Source: CAD feature listing. Evaluate the final solid. Frame: model axes, mm. A direction names the side the tool comes from. Coordinates: 2 decimals unless noted, no trailing zeros. Order: outer loops, then holes, each group sorted by start corner. A loop starts at its lowest first (then second) coordinate and runs counter-clockwise, first axis right, second up. Notation, with made-up numbers: (50.25, 20) -> (80.25, 20) arc R36 ccw to (80.25, 58) -> close; hole circle Ø8 at (-29, 36.25). An arc over 180 degrees is marked (long way). Write item = value, one per line. Start each with the question number.
Item 1: Section query D-D (y = -20). Output: boundary loops of the cut face in (x, z).
Item 2: Set-up query: faces 4 (the cylindrical face through (-0.521, -16.034, 2.535)), 5 (the flat face through (0, 1, 5)). Return all of +Z, -Z, +X, -X, +Y, -Y with unobstructed straight access to the full face (end or side cutting, diameter ignored); none if empty.
Item 3: Section query C-C (x = 9). Output: boundary loops of the cut face in (y, z), then the cut area to 3 significant figures.
Item 4: Contact query for flat-ended pins moving along their axis: pin 1 (1 mm diameter, centred on x = -17, y = 9.5, fed in from -Z); pin 2 (3 mm diameter, centred on x = -5, z = 42, fed in from -Y). Output: stop coordinate, or through.
Item 5: Mould query, pull axis X, two halves, no side actions, for faces 1 (the cylindrical face through (17.482, -32.871, 67.535)), 2 (the cylindrical face through (-0.521, -16.034, 67.535)), 3 (the flat face through (-6, 40, 35)). Classes: released by +X, released by -X, zero draft, split by the parting line, or undercut.
Item 6: Section query A-A (y = -5). Output: boundary loops of the cut face in (x, z), then the cut area to 3 significant figures.
Item 7: Ray query, line 1 along Z through (x, y) = (15, -21); line 2 along Y through (x, z) = (0, 1.65); line 3 along Z through (x, y) = (0, 43). Return the intervals inside material, ascending. Write a range as [from, to].
Item 8: Section query B-B (z = 35). Output: boundary loops of the cut face in (x, y).
```python
from build123d import *

# Parameters (mm, degrees)
SKETCH_1_W          = 50
SKETCH_1_H          = 80
EXTRUDE_1_DEPTH     = 5
SKETCH_2_W          = 50
SKETCH_2_H          = 80
EXTRUDE_2_DEPTH     = 5
SKETCH_3_W          = 50
SKETCH_3_H          = 70
EXTRUDE_3_DEPTH     = 5
SKETCH_4_R          = 4
CUT_EXTRUDE_1_DEPTH = 87.890735985
SKETCH_5_R          = 4
CUT_EXTRUDE_2_DEPTH = 113.915897906
FILLET_1_R          = 25


with BuildPart() as part:
    # Sketch 1 → Extrude 1 (new body)
    with BuildSketch(Plane.XY):
        Rectangle(SKETCH_1_W, SKETCH_1_H)
    extrude(amount=EXTRUDE_1_DEPTH)



with BuildPart() as body_2:
    # Sketch 2 → Extrude 2 (new body)
    with BuildSketch(Plane.XY.offset(65)):
        Rectangle(SKETCH_2_W, SKETCH_2_H)
    extrude(amount=EXTRUDE_2_DEPTH)


with BuildPart() as part_1:
    add(part.part)

    add(body_2.part)  # Extrude 3 merges body 2
    # Sketch 3 → Extrude 3 (add)
    with BuildSketch(Plane(origin=(0, 40, 0), x_dir=(1, 0, 0), z_dir=(0, 1, 0))):
        with Locations((0, -35)):
            Rectangle(SKETCH_3_W, SKETCH_3_H)
    extrude(amount=EXTRUDE_3_DEPTH)

    # Sketch 4 → Cut-Extrude 1 (cut, through all)
    with BuildSketch(Plane.XY.offset(70)):
        with Locations((0, -20)):
            Circle(SKETCH_4_R)
    extrude(amount=-CUT_EXTRUDE_1_DEPTH, mode=Mode.SUBTRACT)

    # Sketch 5 → Cut-Extrude 2 (cut, through all)
    with BuildSketch(Plane(origin=(0, 45, 0), x_dir=(1, 0, 0), z_dir=(0, 1, 0))):
        with Locations(Location((0, -35, 0), (0, 0, 180))):
            Circle(SKETCH_5_R)
    extrude(amount=-CUT_EXTRUDE_2_DEPTH, mode=Mode.SUBTRACT)

    # Fillet 1
    fillet_1_edges = [part_1.edges().sort_by_distance(p)[0] for p in [
        (-25, -40, 2.5),
        (25, -40, 2.5),
        (25, -40, 67.5),
        (-25, -40, 67.5),
    ]]
    fillet(fillet_1_edges, radius=FILLET_1_R - 0.0001)  # a hair under: the kernel refuses the full size


solid = part_1.part
```
Computed:
q1.outline = (-24.49, 0) -> (-4, 0) -> (-4, 5) -> (-24.49, 5) -> close; (-24.49, 65) -> (-4, 65) -> (-4, 70) -> (-24.49, 70) -> close; (4, 0) -> (24.49, 0) -> (24.49, 5) -> (4, 5) -> close; (4, 65) -> (24.49, 65) -> (24.49, 70) -> (4, 70) -> close
q2.face_4 = +Z, -Z
q2.face_5 = +X, -X, -Y
q3.outline = (-38.32, 0) -> (45, 0) -> (45, 70) -> (-38.32, 70) -> (-38.32, 65) -> (40, 65) -> (40, 5) -> (-38.32, 5) -> close
q3.area = 1,130 mm^2
q4.pin_1 = 0
q4.pin_2 = 40
q5.face_1 = released by +X
q5.face_2 = undercut
q5.face_3 = zero draft
q6.outline = (-25, 0) -> (25, 0) -> (25, 5) -> (-25, 5) -> close; (-25, 65) -> (25, 65) -> (25, 70) -> (-25, 70) -> close
q6.area = 500 mm^2
q7.line_1 = [0, 5], [65, 70]
q7.line_2 = [-40, -24], [-16, 45]
q7.line_3 = [0, 31], [39, 70]
q8.outline = (-25, 40) -> (-4, 40) -> (-4, 45) -> (-25, 45) -> close; (4, 40) -> (25, 40) -> (25, 45) -> (4, 45) -> close
